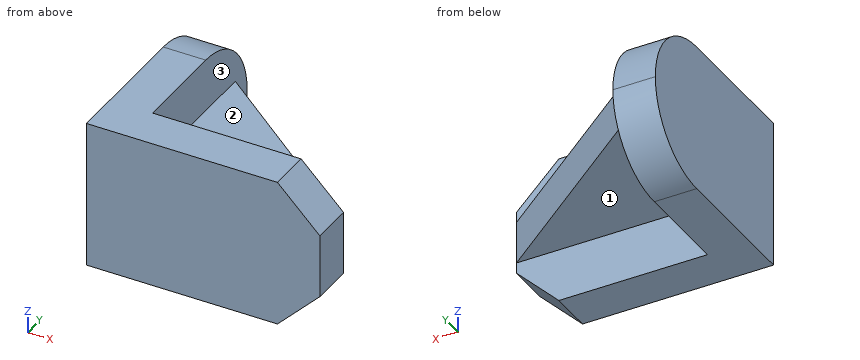
```python
from build123d import *

# Parameters (mm, degrees)
BOSS_EXTRUDE1_DEPTH = 30.48
BOSS_EXTRUDE2_DEPTH = 121.92
SKETCH2_3_W         = 137.16
SKETCH2_3_H         = 30.48
BOSS_EXTRUDE3_DEPTH = 106.68
FILLET1_R           = 53.34
CHAMFER1_SIZE2      = 137.16
CHAMFER1_SIZE       = 106.68


with BuildPart() as part:
    # Sketch1 → Boss-Extrude1 (new body)
    with BuildSketch(Plane(origin=(0, 0, 0), x_dir=(1, 0, 0), z_dir=(0, 1, 0))):
        Polygon((0, 0), (137.16, 0), (167.64, 30.48), (167.64, 76.2), (137.16, 106.68), (0, 106.68), align=None)
    extrude(amount=BOSS_EXTRUDE1_DEPTH)

    # Sketch2 → Boss-Extrude2 (add)
    with BuildSketch(Plane(origin=(0, 30.48, 0), x_dir=(1, 0, 0), z_dir=(0, 1, 0))):
        Polygon((30.48, 106.68), (0, 106.68), (0, 0), (30.48, 0), (30.48, 38.1), (30.48, 68.58), align=None)
    extrude(amount=BOSS_EXTRUDE2_DEPTH)

    # Sketch2<3> → Boss-Extrude3 (add)
    with BuildSketch(Plane(origin=(0, 30.48, 0), x_dir=(1, 0, 0), z_dir=(0, 1, 0))):
        with Locations((99.06, 53.34)):
            Rectangle(SKETCH2_3_W, SKETCH2_3_H)
    extrude(amount=BOSS_EXTRUDE3_DEPTH)

    # Fillet1
    fillet1_edges = [part.edges().sort_by_distance(p)[0] for p in [
        (15.24, 152.4, 0),
        (15.24, 152.4, -106.68),
    ]]
    fillet(fillet1_edges, radius=FILLET1_R - 0.0001)  # a hair under: the kernel refuses the full size

    # Chamfer1
    chamfer1_edges = [part.edges().sort_by_distance(p)[0] for p in [
        (167.64, 137.16, -53.34),
    ]]
    chamfer1_side = [part.faces().sort_by_distance(p)[0] for p in [
        (167.64, 135.0264, -53.34),
    ]]
    chamfer(chamfer1_edges, length=CHAMFER1_SIZE - 0.0001, length2=CHAMFER1_SIZE2 - 0.0001, reference=chamfer1_side[0])  # a hair under: the kernel refuses the full size


solid = part.part
```
The model under review builds one solid part; all positions refer to its coordinate system, in mm. Face numbers are marked on the shaded views. A direction names the side the tool comes from. Round coordinates to 2 decimals unless told otherwise and drop trailing zeros. Loops run counter-clockwise (first coordinate to the right, second up) from the corner with the lowest first, then second, coordinate; pieces in that order, holes last.
1) Tool access review of the marked faces 1, 2 and 3: name each direction out of +Z, -Z, +X, -X, +Y, -Y from which nothing blocks a thin tool from reaching the whole face with its end or side.
Values follow:
face 1: -Z, +X, +Y
face 2: +Z, +X, +Y
face 3: +X, +Y
2) Consider section A-A on x = 80.5. State the section outline as (y, z) points.
Values follow:
outline: (0, -106.68) - (30.48, -106.68) - (30.48, -68.58) - (98.26, -68.58) - (98.26, -38.1) - (30.48, -38.1) - (30.48, 0) - (0, 0) - close
3) Consider section C-C on z = -85. State the section outline as (x, y) points, then the cut area to 3 significant figures.
Values follow:
outline: (0, 0) - (158.84, 0) - (158.84, 30.48) - (30.48, 30.48) - (30.48, 141.99) - (0, 141.99) - close
area: 8,240 mm2
4) Clearance check with flat-ended pins moving along their axes: P1, Ø3, axis at y = 61, z = -62.5, coming from the -X side; P2, Ø1.5, axis at x = 40.5, y = 126, coming from the +Z side; P3, Ø4, axis at y = 36.5, z = -11, coming from the +X side. State where each tip first meets the part, or that it passes through.
Values follow:
P1: stops at x = 0
P2: stops at z = -38.1
P3: stops at x = 30.48
5) Wall thickness on line 1 along Y through (x, z) = (72, -20.5); line 2 along Z through (x, y) = (76, 38.5): over which ranges is each line inside the solid? List them lowest first.
Values follow:
line 1: y = 0 to 30.48
line 2: z = -68.58 to -38.1
6) Consider section B-B on y = 69.5. State the section outline as (x, z) points, then the cut area to 3 significant figures.
Values follow:
outline: (0, -106.68) - (30.48, -106.68) - (30.48, -68.58) - (117.47, -68.58) - (117.47, -38.1) - (30.48, -38.1) - (30.48, 0) - (0, 0) - close
area: 5,900 mm2
